```python
from build123d import *

# Parameters (mm, degrees)
BOSS_EXTRUDE1_DEPTH = 5
FILLET1_R           = 1
FILLET2_R           = 1
BOSS_EXTRUDE2_DEPTH = 5
BOSS_EXTRUDE3_DEPTH = 5
CUT_EXTRUDE1_DEPTH  = 5
BOSS_EXTRUDE4_DEPTH = 5


with BuildPart() as part:
    # Sketch1 → Boss-Extrude1 (new body)
    with BuildSketch(Plane.XY):
        with BuildLine():
            Line((46.328585563, 67.665133516), (48.353724123, 68.117689166))
            ThreePointArc((48.353724123, 68.117689166), (48.398647133, 75.753686317), (47.81637492, 83.367583456))
            Line((47.81637492, 83.367583456), (39.963901457, 81.612799216))
            ThreePointArc((39.963901457, 81.612799216), (40.443341541, 73.963706944), (40.231134371, 66.302542314))
            Line((40.231134371, 66.302542314), (42.267565607, 66.757621526))
            ThreePointArc((42.267565607, 66.757621526), (42.38586051, 68.984034012), (42.447007404, 71.212748282))
            ThreePointArc((42.447007404, 71.212748282), (42.700281141, 71.459795226), (42.452870187, 71.712713391))
            ThreePointArc((42.452870187, 71.712713391), (42.455422518, 72.097266143), (42.4562733, 72.481826424))
            ThreePointArc((42.4562733, 72.481826424), (44.4562733, 74.481826424), (46.4562733, 72.481826424))
            ThreePointArc((46.4562733, 72.481826424), (46.455410169, 72.085672321), (46.452820794, 71.68952574))
            ThreePointArc((46.452820794, 71.68952574), (46.200314758, 71.442404649), (46.447088433, 71.189559074))
            ThreePointArc((46.447088433, 71.189559074), (46.404927274, 69.426771663), (46.328585563, 67.665133516))
        make_face()
    extrude(amount=BOSS_EXTRUDE1_DEPTH)

    # Fillet1
    fillet1_edges = [part.edges().sort_by_distance(p)[0] for p in [
        (46.447088433, 71.189559074, 2.5),
        (46.452820794, 71.68952574, 2.5),
        (42.452870187, 71.712713391, 2.5),
        (42.447007404, 71.212748282, 2.5),
    ]]
    fillet(fillet1_edges, radius=FILLET1_R)

    # Fillet2
    fillet2_edges = [part.edges().sort_by_distance(p)[0] for p in [
        (48.353724123, 68.117689166, 2.5),
        (46.328585563, 67.665133516, 2.5),
        (42.267565607, 66.757621526, 2.5),
        (40.231134371, 66.302542314, 2.5),
    ]]
    fillet(fillet2_edges, radius=FILLET2_R - 0.0001)  # a hair under: the kernel refuses the full size

    # Sketch2 → Boss-Extrude2 (add)
    with BuildSketch(Plane.XY.offset(5)):
        with BuildLine():
            Line((39.70200957, 79.50494448), (38.844189625, 84.436573388))
            Line((38.844189625, 84.436573388), (41.771975747, 85.090842768))
            Line((41.771975747, 85.090842768), (42.426245127, 82.163056646))
            Line((42.426245127, 82.163056646), (40.317359796, 67.626756722))
            ThreePointArc((40.317359796, 67.626756722), (40.333588714, 73.582630469), (39.70200957, 79.50494448))
        make_face()
        with BuildLine():
            Line((48.485367937, 81.467752621), (47.627547992, 86.399381529))
            Line((47.627547992, 86.399381529), (44.699761869, 85.745112148))
            Line((44.699761869, 85.745112148), (45.35403125, 82.817326026))
            Line((45.35403125, 82.817326026), (48.38673347, 68.887746621))
            ThreePointArc((48.38673347, 68.887746621), (48.533086838, 75.176988802), (48.485367937, 81.467752621))
        make_face()
    extrude(amount=-BOSS_EXTRUDE2_DEPTH)

    # Sketch3 → Boss-Extrude3 (add)
    with BuildSketch(Plane.XY.offset(5)):
        with BuildLine():
            ThreePointArc((41.66293085, 85.578807122), (41.961435476, 85.389347393), (41.771975747, 85.090842768))
            Line((41.771975747, 85.090842768), (38.844189625, 84.436573388))
            ThreePointArc((38.844189625, 84.436573388), (38.545685, 84.626033116), (38.735144728, 84.924537741))
            Line((38.735144728, 84.924537741), (41.66293085, 85.578807122))
        make_face()
        with BuildLine():
            ThreePointArc((47.518503095, 86.887345882), (47.81700772, 86.697886154), (47.627547992, 86.399381529))
            Line((47.627547992, 86.399381529), (44.699761869, 85.745112148))
            ThreePointArc((44.699761869, 85.745112148), (44.401257244, 85.934571877), (44.590716973, 86.233076502))
            Line((44.590716973, 86.233076502), (47.518503095, 86.887345882))
        make_face()
    extrude(amount=-BOSS_EXTRUDE3_DEPTH)

    # Sketch4 → Cut-Extrude1 (cut)
    with BuildSketch(Plane.XY.offset(5)):
        Polygon((39.711073435, 85.142627535), (40.365342816, 82.214841413), (41.341271523, 82.432931206), (40.687002143, 85.360717328), align=None)
        Polygon((46.542574388, 86.669256089), (45.56664568, 86.451166295), (46.22091506, 83.523380173), (47.196843768, 83.741469966), align=None)
    extrude(amount=-CUT_EXTRUDE1_DEPTH, mode=Mode.SUBTRACT)

    # Sketch5 → Boss-Extrude4 (add)
    with BuildSketch(Plane.XY.offset(5)):
        with BuildLine():
            Line((39.358881592, 81.477596043), (36.43109547, 80.823326663))
            Line((36.43109547, 80.823326663), (36.649185263, 79.847397955))
            ThreePointArc((36.649185263, 79.847397955), (39.257727558, 77.165710562), (40.333588714, 73.582630469))
            Line((40.333588714, 73.582630469), (44.031942568, 76.908555657))
            Line((44.031942568, 76.908555657), (48.533086838, 75.176988802))
            ThreePointArc((48.533086838, 75.176988802), (49.257403766, 79.374463858), (51.288115875, 83.118744857))
            Line((51.288115875, 83.118744857), (51.070026081, 84.094673564))
            Line((51.070026081, 84.094673564), (48.142239959, 83.440404184))
            Line((48.142239959, 83.440404184), (46.362753702, 81.840114326))
            Line((46.362753702, 81.840114326), (39.358881592, 81.477596043))
        make_face()
    extrude(amount=-BOSS_EXTRUDE4_DEPTH)


solid = part.part
```
Design review of the part built by this model. Coordinates are the model's own, in mm. A direction names the side the tool comes from. Round coordinates to 2 decimals unless told otherwise and drop trailing zeros. Write each loop counter-clockwise with the first axis right and the second up, starting at its lowest first coordinate (ties: lowest second). Pieces come first, ordered by that corner, then holes. Notation, with made-up numbers: (65, -0.5) -> (123, -0.5) arc R29 cw to (123, 23.5) -> close; hole circle Ø8 at (6.5, -11.5). An arc over 180 degrees is marked (long way). Answer in a Markdown table with one row per item.
Q1. Draft analysis for pull direction X (two halves, no side actions). For faces 1 (the face through (48.16, 68.29, 2.54)), 2 (the face through (45.07, 86.34, 2.54)), 3 (the face through (42.095, 83.647, 2.535)), state which applies: +X half, -X half, draft (parallel to the pull), parting line (faces both ways), or undercut.
The answers:
| item | result |
|---|---|
| face 1 | +X half |
| face 2 | -X half |
| face 3 | undercut |
Q2. Take a section at A-A, the plane y = 69.5. State the section outline as (x, z) points.
The answers:
| item | result |
|---|---|
| outline | (40.39, 0) -> (42.41, 0) -> (42.41, 5) -> (40.39, 5) -> close; (46.41, 0) -> (48.41, 0) -> (48.41, 5) -> (46.41, 5) -> close |
Q3. Take a section at C-C, the plane y = 73.25. State the section outline as (x, z) points, then the cut area to 3 significant figures.
The answers:
| item | result |
|---|---|
| outline | (40.35, 0) -> (42.61, 0) -> (42.61, 5) -> (40.35, 5) -> close; (46.3, 0) -> (48.51, 0) -> (48.51, 5) -> (46.3, 5) -> close |
| area | 22.3 mm² |
Q4. To check wall thickness, follow L1, parallel to X at y = 84.5, z = 2.2; L2, parallel to X at y = 85.25, z = 1.7; L3, parallel to X at y = 83, z = 3.35. State the ranges of each line that lie inside material, in increasing order. Write a range as [from, to].
The answers:
| item | result |
|---|---|
| L1 | [38.62, 39.85], [40.88, 41.9], [44.98, 46], [47.03, 47.96] |
| L2 | [40.71, 41.95], [44.81, 45.84], [46.86, 47.83] |
| L3 | [39.09, 40.19], [41.21, 42.24], [45.31, 51.2] |
Q5. Take a section at B-B, the plane x = 49. State the section outline as (y, z) points.
The answers:
| item | result |
|---|---|
| outline | (78.54, 0) -> (83.63, 0) -> (83.63, 5) -> (78.54, 5) -> close |
Q6. For faces 4 (the face through (47.89, 84.9, 2.54)), 5 (the face through (49.627, 83.772, 2.535)), 6 (the face through (48.483, 71.988, 2.535)), 7 (the face through (47.024, 86.777, 2.535)), 8 (the face through (39.105, 82.936, 2.535)), list the 3-axis set-ups (+Z, -Z, +X, -X, +Y, -Y) from which the entire face can be reached by the end or side of a thin tool; tool diameter is ignored.
The answers:
| item | result |
|---|---|
| face 4 | +Z, -Z |
| face 5 | +Z, -Z, +Y |
| face 6 | +Z, -Z, +X, -Y |
| face 7 | +Z, -Z, -X, +Y |
| face 8 | +Z, -Z, -X |
Q7. Take a section at D-D, the plane y = 76.75. State the section outline as (x, z) points.
The answers:
| item | result |
|---|---|
| outline | (39.49, 0) -> (48.64, 0) -> (48.64, 5) -> (39.49, 5) -> close |
Q8. Clearance check with flat-ended pins moving along their axes: pin 1 Ø1 at (y, z) = (80, 1) entering from +X; pin 2 Ø1.5 at (y, z) = (84.5, 3.5) entering from +X. State where each tip first meets the part, or that it passes through.
The answers:
| item | result |
|---|---|
| pin 1 | x = 49.71 |
| pin 2 | x = 51.15 |
